Source: three-view drawing plus pictorial views. Frame: mm from the lowest corner of the part. A direction names the side the tool comes from. Give positions to 0.01 mm unless a question says otherwise; leave off trailing zeros. Order: outer loops, then holes, each group sorted by start corner. A loop starts at its lowest first (then second) coordinate and runs counter-clockwise, first axis right, second up. Notation, with made-up numbers: M 17.25,48 L 71.25,48 A27 ccw 71.25,64 Z; hole C -34.5,78.25 d8. An arc over 180 degrees is marked long. Use CSV: the item, a comma, the result in double quotes. Start each with the question number.
Item 1: Pull-direction query (X, two-part tool) for the marked faces 1, 2, 3 and 4; classes: +X half, -X half, draft (parallel to the pull), parting line (faces both ways), or undercut.
Item 2: Section query C-C on z = 342.5. Return loops of the section in (x, y), and give its area (3 significant figures).
Item 3: First-contact query: pin 1 (5 mm diameter, centred on x = 118, y = 570.5, fed in from +Z); pin 2 (8 mm diameter, centred on x = 431.5, z = 327, fed in from +Y); pin 3 (6 mm diameter, centred on y = 399.5, z = 174.5, fed in from -X). Flat tips, straight axial feed; report the tip coordinate or a pass-through.
Item 4: Access query for the marked faces 5 and 6. Directions: +Z, -Z, +X, -X, +Y, -Y. A direction counts if a zero-diameter tool reaches every point of the face in a straight line with its end or side. Return the directions, or none.
Item 5: Section query B-B on y = 504. Return loops of the section in (x, z).
Item 6: Section query D-D on y = 633.5. Return loops of the section in (x, z), and give its area (3 significant figures).
Item 7: Ray query, probe 1 along X at (y, z) = (720, 115.5); probe 2 along Z at (x, y) = (532, 358.5); probe 3 along Y at (x, z) = (640, 209.5). Return the intervals inside material, ascending. Write a range as from..to.
Item 8: Section query A-A on x = 381. Return loops of the section in (y, z), and give its area (3 significant figures).
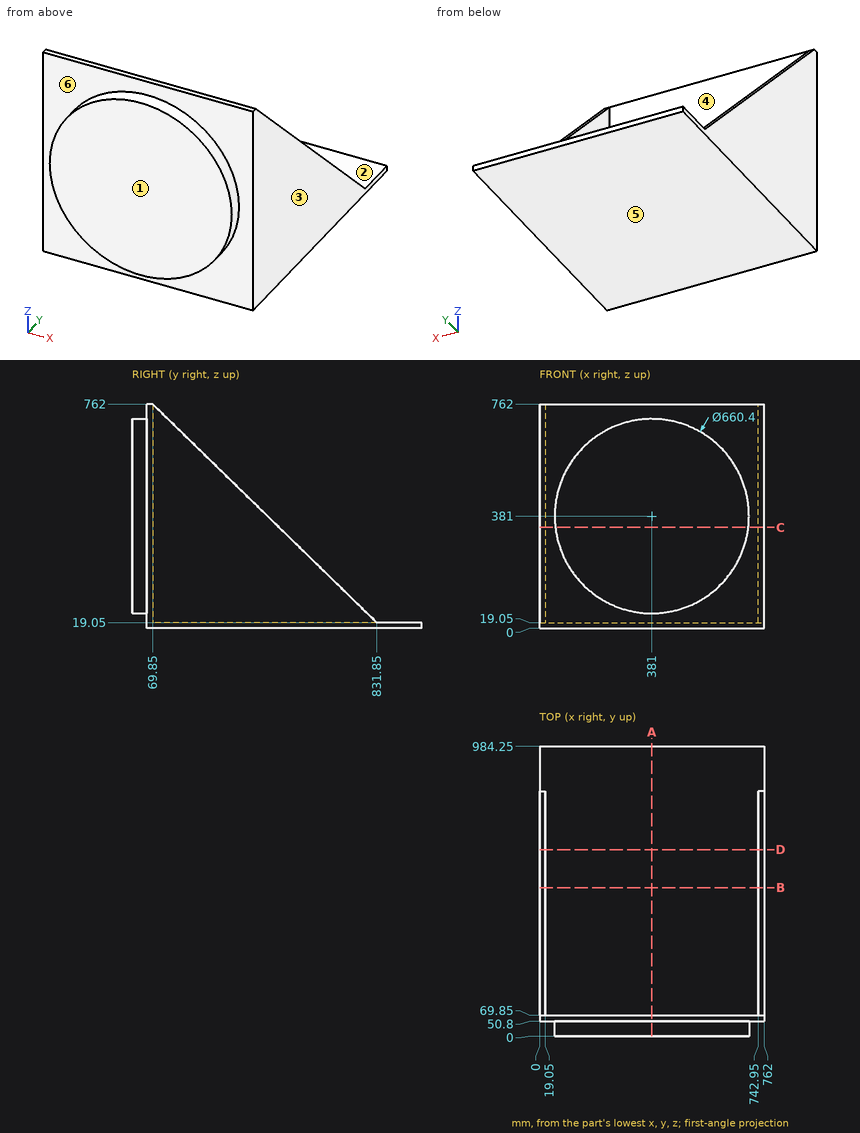
Verdict:
1,face 1,"draft"
1,face 2,"undercut"
1,face 3,"+X half"
1,face 4,"undercut"
2,outline,"M 0,50.8 L 53.05,50.8 L 53.05,0 L 708.95,0 L 708.95,50.8 L 762,50.8 L 762,500.11 L 742.95,500.11 L 742.95,69.85 L 19.05,69.85 L 19.05,500.11 L 0,500.11 Z"
2,area,"64,200 mm2"
3,pin 1,"z = 19.05"
3,pin 2,"y = 69.85"
3,pin 3,"x = 0"
4,face 5,"-Z, +X, -X, +Y, -Y"
4,face 6,"-Y"
5,outline,"M 0,0 L 762,0 L 762,338.7 L 742.95,338.7 L 742.95,19.05 L 19.05,19.05 L 19.05,338.7 L 0,338.7 Z"
6,outline,"M 0,0 L 762,0 L 762,212.44 L 742.95,212.44 L 742.95,19.05 L 19.05,19.05 L 19.05,212.44 L 0,212.44 Z"
6,area,"21,900 mm2"
7,probe 1,"0..19.05, 742.95..762"
7,probe 2,"0..19.05"
7,probe 3,"0..69.85"
8,outline,"M 0,50.8 L 50.8,50.8 L 50.8,0 L 984.25,0 L 984.25,19.05 L 69.85,19.05 L 69.85,762 L 50.8,762 L 50.8,711.2 L 0,711.2 Z"
8,area,"65,500 mm2"
